Check sheet for the modelled part. Datum: model origin and axes. Units: mm. A direction names the side the tool comes from. Coordinates: 2 decimals unless noted, no trailing zeros. Loops run counter-clockwise (first coordinate to the right, second up) from the corner with the lowest first, then second, coordinate; pieces in that order, holes last. Notation, with made-up numbers: (-39.5, 68.25) - (-34.5, 68.25) arc R27 ccw to (-34.5, 99.25) - close; hole circle Ø5 at (-4, -21). An arc over 180 degrees is marked (long way). Use a Markdown table: item, result. Add a question column.
1) Thickness scan on line 1 (Y direction, x = 28.5, z = 24.2); line 2 (Y direction, x = 21.5, z = -17); line 3 (Z direction, x = 13, y = 16.5). Record the ranges inside material, lowest first.
2) Go/stop test with flat-tipped pins: P1, Ø1.2, axis at x = 29, y = 8.5, coming from the -Z side; P2, Ø4, axis at y = 25, z = 19, coming from the -X side; P3, Ø4.5, axis at x = 15.5, z = -10, coming from the -Y side; P4, Ø6.5, axis at x = 10.5, y = 8, coming from the -Z side. Record where each tip stops, or that it passes through.
3) Tool access check on faces 4 (the flat face through (35.8, 17, -14)), 5 (the flat face through (19, 30.8, -14)), 6 (the cylindrical face through (12.1, 27.2, 24.5)), 7 (the flat face through (20, 2.4, -6)), 8 (the cylindrical face through (30.347, 26.766, -22.493)). Record the directions out of +Z, -Z, +X, -X, +Y, -Y that give a thin tool (end or side, any length) a straight path to the whole face; none if there is none.
4) Sectioned sample at B-B, the plane y = 11.5. Enter the section's corners in (x, z), then the cut area to 3 significant figures.
5) Draft check along Y on faces 1 (the cylindrical face through (25.55, 19.7, 24.51)), 2 (the flat face through (0, 17, 11)), 3 (the flat face through (-1, 7, -11)). Enter one of: pulls with the +Y half, pulls with the -Y half, needs draft (parallel to the pull), parting line crosses it, or undercut.
6) Sectioned sample at A-A, the plane z = -13.5. Enter the section's corners in (x, y).
7) Sectioned sample at C-C, the plane z = 5. Enter the section's corners in (x, y).
8) Sectioned sample at D-D, the plane z = 16.5. Enter the section's corners in (x, y), then the cut area to 3 significant figures.
from build123d import *

# Parameters (mm, degrees)
EXTRUDE_1_DEPTH     = 25
EXTRUDE_3_DEPTH     = 4
EXTRUDE_4_DEPTH     = 4
EXTRUDE_5_DEPTH     = 4
EXTRUDE_6_DEPTH     = 4
EXTRUDE_7_DEPTH     = 7
SKETCH_7_W          = 23
SKETCH_7_H          = 20
EXTRUDE_8_DEPTH     = 8.5
SKETCH_8_W          = 16.231712275
SKETCH_8_H          = 15.860541866
EXTRUDE_9_DEPTH     = 3
FILLET_1_R          = 3
FILLET_2_R          = 1
SKETCH_9_R          = 4
SKETCH_9_R_2        = 2
CUT_EXTRUDE_1_DEPTH = 1
CUT_EXTRUDE_START   = -1
SKETCH_10_R         = 4
SKETCH_10_R_2       = 2
CUT_EXTRUDE_2_DEPTH = 1


with BuildPart() as part:
    # ｽｹｯﾁ1 → ﾎﾞｽ - 押し出し1 (new body)
    with BuildSketch(Plane.XY):
        with BuildLine():
            Line((7, 0), (32, 0))
            ThreePointArc((32, 0), (36.949747468, 2.050252532), (39, 7))
            Line((39, 7), (39, 27))
            ThreePointArc((39, 27), (36.949747468, 31.949747468), (32, 34))
            Line((32, 34), (7, 34))
            ThreePointArc((7, 34), (2.050252532, 31.949747468), (0, 27))
            Line((0, 27), (0, 7))
            ThreePointArc((0, 7), (2.050252532, 2.050252532), (7, 0))
        make_face()
    extrude(amount=EXTRUDE_1_DEPTH)

    # ｽｹｯﾁ2 → ﾎﾞｽ - 押し出し3 (add)
    with BuildSketch(Plane(origin=(0, 0, 0), x_dir=(-1, 0, 0), z_dir=(0, 0, -1))):
        with BuildLine():
            Line((-37, 27), (-37, 7))
            ThreePointArc((-37, 7), (-35.535533906, 3.464466094), (-32, 2))
            Line((-32, 2), (-7, 2))
            ThreePointArc((-7, 2), (-3.464466094, 3.464466094), (-2, 7))
            Line((-2, 7), (-2, 27))
            ThreePointArc((-2, 27), (-3.464466094, 30.535533906), (-7, 32))
            Line((-7, 32), (-32, 32))
            ThreePointArc((-32, 32), (-35.535533906, 30.535533906), (-37, 27))
        make_face()
    extrude(amount=EXTRUDE_3_DEPTH)

    # ｽｹｯﾁ3 → ﾎﾞｽ - 押し出し4 (add)
    with BuildSketch(Plane(origin=(0, 0, -4), x_dir=(-1, 0, 0), z_dir=(0, 0, -1))):
        with BuildLine():
            Line((-32, 2.4), (-7, 2.4))
            ThreePointArc((-7, 2.4), (-3.747308807, 3.747308807), (-2.4, 7))
            Line((-2.4, 7), (-2.4, 27))
            ThreePointArc((-2.4, 27), (-3.747308807, 30.252691193), (-7, 31.6))
            Line((-7, 31.6), (-32, 31.6))
            ThreePointArc((-32, 31.6), (-35.252691193, 30.252691193), (-36.6, 27))
            Line((-36.6, 27), (-36.6, 7))
            ThreePointArc((-36.6, 7), (-35.252691193, 3.747308807), (-32, 2.4))
        make_face()
    extrude(amount=EXTRUDE_4_DEPTH)

    # ｽｹｯﾁ4 → ﾎﾞｽ - 押し出し5 (add)
    with BuildSketch(Plane(origin=(0, 0, -8), x_dir=(-1, 0, 0), z_dir=(0, 0, -1))):
        with BuildLine():
            Line((-36.2, 27), (-36.2, 7))
            ThreePointArc((-36.2, 7), (-34.969848481, 4.030151519), (-32, 2.8))
            Line((-32, 2.8), (-7, 2.8))
            ThreePointArc((-7, 2.8), (-4.030151519, 4.030151519), (-2.8, 7))
            Line((-2.8, 7), (-2.8, 27))
            ThreePointArc((-2.8, 27), (-4.030151519, 29.969848481), (-7, 31.2))
            Line((-7, 31.2), (-32, 31.2))
            ThreePointArc((-32, 31.2), (-34.969848481, 29.969848481), (-36.2, 27))
        make_face()
    extrude(amount=EXTRUDE_5_DEPTH)

    # ｽｹｯﾁ5 → ﾎﾞｽ - 押し出し6 (add)
    with BuildSketch(Plane(origin=(0, 0, -12), x_dir=(-1, 0, 0), z_dir=(0, 0, -1))):
        with BuildLine():
            Line((-35.8, 27), (-35.8, 7))
            ThreePointArc((-35.8, 7), (-34.687005769, 4.312994231), (-32, 3.2))
            Line((-32, 3.2), (-7, 3.2))
            ThreePointArc((-7, 3.2), (-4.312994231, 4.312994231), (-3.2, 7))
            Line((-3.2, 7), (-3.2, 27))
            ThreePointArc((-3.2, 27), (-4.312994231, 29.687005769), (-7, 30.8))
            Line((-7, 30.8), (-32, 30.8))
            ThreePointArc((-32, 30.8), (-34.687005769, 29.687005769), (-35.8, 27))
        make_face()
    extrude(amount=EXTRUDE_6_DEPTH)

    # ｽｹｯﾁ6 → ﾎﾞｽ - 押し出し7 (add)
    with BuildSketch(Plane(origin=(0, 0, -16), x_dir=(-1, 0, 0), z_dir=(0, 0, -1))):
        with BuildLine():
            Line((-35.4, 27), (-35.4, 7))
            ThreePointArc((-35.4, 7), (-34.404163056, 4.595836944), (-32, 3.6))
            Line((-32, 3.6), (-7, 3.6))
            ThreePointArc((-7, 3.6), (-4.595836944, 4.595836944), (-3.6, 7))
            Line((-3.6, 7), (-3.6, 27))
            ThreePointArc((-3.6, 27), (-4.595836944, 29.404163056), (-7, 30.4))
            Line((-7, 30.4), (-32, 30.4))
            ThreePointArc((-32, 30.4), (-34.404163056, 29.404163056), (-35.4, 27))
        make_face()
    extrude(amount=EXTRUDE_7_DEPTH)

    # ｽｹｯﾁ7 → ﾎﾞｽ - 押し出し8 (add)
    with BuildSketch(Plane.ZY.offset(-3.6)):
        with Locations((-11.5, 17)):
            Rectangle(SKETCH_7_W, SKETCH_7_H)
    extrude(amount=EXTRUDE_8_DEPTH)

    # ｽｹｯﾁ8 → ﾎﾞｽ - 押し出し9 (add)
    with BuildSketch(Plane(origin=(39, 0, 0), x_dir=(0, 0, -1), z_dir=(1, 0, 0))):
        with Locations((-16.884143863, 17.283223962)):
            Rectangle(SKETCH_8_W, SKETCH_8_H)
    extrude(amount=EXTRUDE_9_DEPTH)

    # ﾌｨﾚｯﾄ1
    fillet_1_edges = [part.edges().sort_by_distance(p)[0] for p in [
        (39, 26.106747447, 25),
        (40.5, 25.213494895, 25),
        (42, 17.283223962, 25),
        (40.5, 9.352953029, 25),
        (39, 8.176476514, 25),
        (36.949747468, 2.050252532, 25),
        (19.5, 0, 25),
        (2.050252532, 2.050252532, 25),
        (0, 17, 25),
        (2.050252532, 31.949747468, 25),
        (19.5, 34, 25),
        (36.949747468, 31.949747468, 25),
    ]]
    fillet(fillet_1_edges, radius=FILLET_1_R)

    # ﾌｨﾚｯﾄ2
    fillet_2_edges = [part.edges().sort_by_distance(p)[0] for p in [
        (34.404163056, 29.404163056, -23),
        (35.4, 17, -23),
        (34.404163056, 4.595836944, -23),
        (19.5, 3.6, -23),
        (4.595836944, 4.595836944, -23),
        (4.595836944, 29.404163056, -23),
        (19.5, 30.4, -23),
        (-0.65, 7, -23),
        (-0.65, 27, -23),
        (-4.9, 17, -23),
    ]]
    fillet(fillet_2_edges, radius=FILLET_2_R)

    # ｽｹｯﾁ9 → ｶｯﾄ - 押し出し1 (cut)
    with BuildSketch(Plane.XY.offset(25)):
        with Locations((19.5, 17)):
            Circle(SKETCH_9_R)
        with Locations((28.5, 17)):
            Circle(SKETCH_9_R)
        with Locations(Location((10.5, 17, 0), (0, 0, 180))):
            Circle(SKETCH_9_R)
        with Locations((16.5, 8)):
            Circle(SKETCH_9_R_2)
        with Locations((10.5, 8)):
            Circle(SKETCH_9_R_2)
        with Locations(Location((22.5, 8, 0), (0, 0, 180))):
            Circle(SKETCH_9_R_2)
        with Locations(Location((28.5, 8, 0), (0, 0, 180))):
            Circle(SKETCH_9_R_2)
        with Locations((28.5, 26)):
            Circle(SKETCH_9_R_2)
        with Locations((22.5, 26)):
            Circle(SKETCH_9_R_2)
        with Locations(Location((16.5, 26, 0), (0, 0, 180))):
            Circle(SKETCH_9_R_2)
        with Locations(Location((10.5, 26, 0), (0, 0, 180))):
            Circle(SKETCH_9_R_2)
    extrude(amount=-CUT_EXTRUDE_1_DEPTH, mode=Mode.SUBTRACT)

    # ｽｹｯﾁ10 → ｶｯﾄ - 押し出し2 (cut)
    with BuildSketch(Plane(origin=(0, 0, -23), x_dir=(-1, 0, 0), z_dir=(0, 0, -1)).offset(CUT_EXTRUDE_START)):
        with Locations(Location((-19.5, 17, 0), (0, 0, 180))):
            Circle(SKETCH_10_R)
        with Locations((-10.5, 17)):
            Circle(SKETCH_10_R)
        with Locations(Location((-28.5, 17, 0), (0, 0, 180))):
            Circle(SKETCH_10_R)
        with Locations((-16.5, 26)):
            Circle(SKETCH_10_R_2)
        with Locations((-10.5, 26)):
            Circle(SKETCH_10_R_2)
        with Locations(Location((-28.5, 26, 0), (0, 0, 180))):
            Circle(SKETCH_10_R_2)
        with Locations(Location((-22.5, 26, 0), (0, 0, 180))):
            Circle(SKETCH_10_R_2)
        with Locations(Location((-10.5, 8, 0), (0, 0, 180))):
            Circle(SKETCH_10_R_2)
        with Locations(Location((-16.5, 8, 0), (0, 0, 180))):
            Circle(SKETCH_10_R_2)
        with Locations((-22.5, 8)):
            Circle(SKETCH_10_R_2)
        with Locations((-28.5, 8)):
            Circle(SKETCH_10_R_2)
    extrude(amount=CUT_EXTRUDE_2_DEPTH, mode=Mode.SUBTRACT)


solid = part.part
Solved:
| question | item | result |
|---|---|---|
| 1 | line 1 | y = 0.96 to 6, 10 to 13, 21 to 24, 28 to 33.04 |
| 1 | line 2 | y = 3.6 to 30.4 |
| 1 | line 3 | z = -22 to 24 |
| 2 | P1 | stops at z = -22 |
| 2 | P2 | stops at x = 0 |
| 2 | P3 | stops at y = 2.4 |
| 2 | P4 | stops at z = -23 |
| 3 | face 4 | -Z, +X, +Y, -Y |
| 3 | face 5 | -Z, +X, -X, +Y |
| 3 | face 6 | +Z |
| 3 | face 7 | -Z, +X, -X, -Y |
| 3 | face 8 | -Z |
| 4 | outline | (-4.9, -22) arc R1 ccw to (-3.9, -23) - (34.4, -23) arc R1 ccw to (35.4, -22) - (35.4, -16) - (35.8, -16) - (35.8, -12) - (36.2, -12) - (36.2, -8) - (36.6, -8) - (36.6, -4) - (37, -4) - (37, 0) - (39, 0) - (39, 8.77) - (42, 8.77) - (42, 22) arc R3 ccw to (39.85, 24.88) - (36.85, 24.88) arc R3 ccw to (36, 25) - (3, 25) arc R3 ccw to (0, 22) - (0, 0) - (-4.9, 0) - close |
| 4 | area | 1,960 mm2 |
| 5 | face 1 | undercut |
| 5 | face 2 | needs draft |
| 5 | face 3 | pulls with the -Y half |
| 6 | outline | (-4.9, 7) - (3.2, 7) arc R3.8 ccw to (7, 3.2) - (32, 3.2) arc R3.8 ccw to (35.8, 7) - (35.8, 27) arc R3.8 ccw to (32, 30.8) - (7, 30.8) arc R3.8 ccw to (3.2, 27) - (-4.9, 27) - close |
| 7 | outline | (0, 7) arc R7 ccw to (7, 0) - (32, 0) arc R7 ccw to (39, 7) - (39, 27) arc R7 ccw to (32, 34) - (7, 34) arc R7 ccw to (0, 27) - close |
| 8 | outline | (0, 7) arc R7 ccw to (7, 0) - (32, 0) arc R7 ccw to (39, 7) - (39, 9.35) - (42, 9.35) - (42, 25.21) - (39, 25.21) - (39, 27) arc R7 ccw to (32, 34) - (7, 34) arc R7 ccw to (0, 27) - close |
| 8 | area | 1,330 mm2 |
